Check sheet for the modelled part. Datum: model origin and axes. Units: mm. A direction names the side the tool comes from. Round coordinates to 2 decimals unless told otherwise and drop trailing zeros. Write each loop counter-clockwise with the first axis right and the second up, starting at its lowest first coordinate (ties: lowest second). Pieces come first, ordered by that corner, then holes. Notation, with made-up numbers: (17.25, 47) - (22.25, 47) arc R23 ccw to (22.25, 55) - close; hole circle Ø3 at (2, -31). An arc over 180 degrees is marked (long way). Use one line per item in the form item = value. Start each with the question number.
1) Section check B-B (x = 0). Record the boundary of the cut face in (y, z), then the cut area to 3 significant figures.
2) Set-up check for faces 1 (the face through (-0.9, 16.24, -2.86)), 2 (the face through (-13.59, -0.14, -43.16)): record each of +Z, -Z, +X, -X, +Y, -Y from which the full face is reachable in a straight line by a thin tool's end or side.
3) Section check C-C (y = 6). Record the boundary of the cut face in (x, z), then the cut area to 3 significant figures.
4) Scan lines: probe 1 along Y at (x, z) = (10, -2); probe 2 along X at (y, z) = (9.5, 1); probe 3 along X at (y, z) = (-6.5, 33). Record each from-to range of solid material in increasing order.
5) Section check A-A (z = 0). Record the boundary of the cut face in (x, y).
6) Gauge pin test, flat ends, axial feed: P1, Ø12, axis at x = -22.5, y = 0.5, coming from the +Z side; P2, Ø1, axis at x = -20.5, y = -4, coming from the +Z side; P3, Ø3, axis at x = 35, y = 4.5, coming from the +Z side. Record the tip position at first contact, or that the pin passes through.
from build123d import *

# Parameters (mm, degrees)
ESQUISSE2_R        = 3
BOSS_EXTRU_1_DEPTH = 2


with BuildPart() as part:
    # Esquisse1 → Révolution1 (revolve)
    with BuildSketch(Plane.XY, mode=Mode.PRIVATE) as r_volution1_sk:
        Polygon((0, 15.25), (-35.25, 15.25), (-45.25, 10.25), (-45.25, -10.25), (-35.25, -15.25), (0, -15.25), align=None)
    revolve(r_volution1_sk.sketch.rotate(Axis((0, -78.381633957, 0), (0, 1, 0)), 270), axis=Axis((0, -78.381633957, 0), (0, 1, 0)))

    # Esquisse2 → Boss.-Extru.1 (add)
    with BuildSketch(Plane(origin=(0, 15.25, 0), x_dir=(1, 0, 0), z_dir=(0, 1, 0))):
        with Locations(Location((0, 0, 0), (0, 0, 90))):
            Circle(ESQUISSE2_R)
    extrude(amount=BOSS_EXTRU_1_DEPTH)


solid = part.part
Results are:
q1.outline = (-15.25, -35.25) - (-10.25, -45.25) - (10.25, -45.25) - (15.25, -35.25) - (15.25, -3) - (17.25, -3) - (17.25, 3) - (15.25, 3) - (15.25, 35.25) - (10.25, 45.25) - (-10.25, 45.25) - (-15.25, 35.25) - close
q1.area = 2,670 mm²
q2.face_1 = +Y
q2.face_2 = +Y, -Y
q3.outline = circle Ø90.5 at (0, 0)
q3.area = 6,430 mm²
q4.probe_1 = -15.25 to 15.25
q4.probe_2 = -45.24 to 45.24
q4.probe_3 = -30.96 to 30.96
q5.outline = (-45.25, -10.25) - (-35.25, -15.25) - (35.25, -15.25) - (45.25, -10.25) - (45.25, 10.25) - (35.25, 15.25) - (3, 15.25) - (3, 17.25) - (-3, 17.25) - (-3, 15.25) - (-35.25, 15.25) - (-45.25, 10.25) - close
q6.P1 = 42.13
q6.P2 = 40.59
q6.P3 = 30.42
